Work out the finished part from the listing and answer in its coordinate system (mm). A direction names the side the tool comes from. Coordinates: 2 decimals unless noted, no trailing zeros. Order: outer loops, then holes, each group sorted by start corner. A loop starts at its lowest first (then second) coordinate and runs counter-clockwise, first axis right, second up.
Autodesk Inventor part; units mm, degrees
ref_plane "YZ Plane" through (0, 0, 0) normal (1, 0, 0) x (0, 1, 0)
ref_plane "XZ Plane" through (0, 0, 0) normal (0, 1, 0) x (-1, 0, 0)
ref_plane "XY Plane" through (0, 0, 0) normal (0, 0, 1) x (1, 0, 0)
sketch "Sketch1" plane through (0, 0, 0) normal (0, 1, 0) x (-1, 0, 0)
  line L0 (27.5, 36) -> (-27.5, 36)
  line L1 (-27.5, 36) -> (-27.5, -36)
  line L2 (-27.5, -36) -> (27.5, -36)
  line L3 (27.5, -36) -> (27.5, 36)
  line L4 (27.5, 36) -> (-27.5, -36) construction
  line L5 (-27.5, 36) -> (27.5, -36) construction
  point P0 (0, 0)
  dimension "d0" = 55
  dimension "d1" = 72
extrude "Extrusion1" add sketch "Sketch1" along normal blind 1.3
sketch "Sketch2" plane through (0, 1.3, 0) normal (0, 1, 0) x (1, 0, 0)
  line L0 (-25, 35) -> (25, 35)
  line L1 (25, 35) -> (25, -35)
  line L2 (25, -35) -> (-25, -35)
  line L3 (-25, -35) -> (-25, 35)
  line L4 (-25, 35) -> (25, -35) construction
  line L5 (25, 35) -> (-25, -35) construction
  point P0 (0, 0)
  dimension "d4" = 70
  dimension "d5" = 50
extrude "Extrusion2" add sketch "Sketch2" along normal blind 4
sketch "Sketch3" plane through (0, 0, 0) normal (0, -1, 0) x (1, 0, 0)
  line L0 (-27.5, -17) -> (-22.5, -17)
  line L1 (-22.5, -17) -> (-22.5, 13)
  line L2 (-22.5, 13) -> (-27.5, 13)
  line L3 (-27.5, 13) -> (-27.5, -17)
  line L4 (27.5, -36) -> (-27.5, -36)
  line L5 (-27.5, -36) -> (-27.5, 36)
  point P0 (0, 0)
  dimension "d8" = 30
  dimension "d9" = 5
  dimension "d10" = 19
  dimension "d11" = 0
extrude "Extrusion3" add sketch "Sketch3" along normal blind 13
properties part number "display"
1. For faces 1 (the flat face through (-25, -6, -17)), 2 (the flat face through (25, 3, 0)), 3 (the flat face through (0, 3, -35)), 4 (the flat face through (-25, 3, 0)), determine the directions among +Z, -Z, +X, -X, +Y, -Y from which every point of the face is accessible in a straight line to the end or side of a thin tool.
2. Flat-ended cylindrical pins translate along their axes: pin 1 (4 mm diameter, centred on y = 3.5, z = 20.5, fed in from -X); pin 2 (2.5 mm diameter, centred on x = -26, y = -7, fed in from -Z); pin 3 (2.5 mm diameter, centred on x = -25.5, y = -4, fed in from +Z); pin 4 (3 mm diameter, centred on x = -19.5, y = -5.5, fed in from +Z). Find the tip coordinate at first contact, or state that the pin passes through.
3. The part is cut by section D-D (z = -23.5). Determine the outline of the cut face in (x, y), plus the area to 4 significant figures.
4. The part is cut by section B-B (z = 4.5). Determine the outline of the cut face in (x, y), plus the area to 4 significant figures.
5. The part is cut by section C-C (y = -6.25). Determine the outline of the cut face in (x, z).
6. Consider probe 1 along Y at (x, z) = (6, 2); probe 2 along X at (y, z) = (-3.5, 0); probe 3 along X at (y, z) = (4, 2). Determine where each line is inside the solid, lowest interval first.
7. The part is cut by section A-A (x = 22). Determine the outline of the cut face in (y, z), plus the area to 3 significant figures.
Worked out:
1. face 1: -Z, +X, -X, -Y
1. face 2: +Z, -Z, +X, +Y
1. face 3: -Z, +X, -X, +Y
1. face 4: +Z, -Z, -X, +Y
2. pin 1: stops at x = -25
2. pin 2: stops at z = -17
2. pin 3: stops at z = 13
2. pin 4: passes through
3. outline: (-27.5, 0) - (27.5, 0) - (27.5, 1.3) - (25, 1.3) - (25, 5.3) - (-25, 5.3) - (-25, 1.3) - (-27.5, 1.3) - close
3. area: 271.5 mm2
4. outline: (-27.5, -13) - (-22.5, -13) - (-22.5, 0) - (27.5, 0) - (27.5, 1.3) - (25, 1.3) - (25, 5.3) - (-25, 5.3) - (-25, 1.3) - (-27.5, 1.3) - close
4. area: 336.5 mm2
5. outline: (-27.5, -17) - (-22.5, -17) - (-22.5, 13) - (-27.5, 13) - close
6. probe 1: y = 0 to 5.3
6. probe 2: x = -27.5 to -22.5
6. probe 3: x = -25 to 25
7. outline: (0, -36) - (1.3, -36) - (1.3, -35) - (5.3, -35) - (5.3, 35) - (1.3, 35) - (1.3, 36) - (0, 36) - close
7. area: 374 mm2
